Can you work these out from the model? Positions are in its coordinate system, mm. Face numbers are marked on the shaded views. Give positions to 0.01 mm unless a question says otherwise; leave off trailing zeros. Loops run counter-clockwise (first coordinate to the right, second up) from the corner with the lowest first, then second, coordinate; pieces in that order, holes last.
from build123d import *

# Parameters (mm, degrees)
BOSS_EXTRUDE1_DEPTH       = 2.54
F_3_0MM_DOWEL_HOLE1_D     = 3
F_3_0MM_DOWEL_HOLE1_DEPTH = 7.999984
F_3_0MM_DOWEL_HOLE1_TIP   = 0.901290929


with BuildPart() as part:
    # Sketch1 → Boss-Extrude1 (new body)
    with BuildSketch(Plane(origin=(0, 0, 0), x_dir=(1, 0, 0), z_dir=(0, 1, 0))):
        Polygon((59.944, 42.386808891), (42.386808891, 59.944), (17.557191109, 59.944), (0, 42.386808891), (0, 17.557191109), (17.557191109, 0), (42.386808891, 0), (59.944, 17.557191109), align=None)
        Polygon((4.468072616, 46.495671263), (6.26412384, 44.699620039), (15.244379961, 53.67987616), (13.448328737, 55.475927384), align=None, mode=Mode.SUBTRACT)
        Polygon((53.67987616, 44.699620039), (44.699620039, 53.67987616), (46.495671263, 55.475927384), (55.475927384, 46.495671263), align=None, mode=Mode.SUBTRACT)
    extrude(amount=BOSS_EXTRUDE1_DEPTH)

    # Ø3.0mm Dowel Hole1
    with Locations(Plane(origin=(0, 2.54, 0), x_dir=(1, 0, 0), z_dir=(0, 1, 0))):
        with Locations((2.9, 18.758410439), (57.044, 18.758410439), (2.9, 41.18558956), (57.044, 41.185589561), (18.758410439, 57.044), (41.185589561, 57.044)):
            Hole(F_3_0MM_DOWEL_HOLE1_D / 2, depth=F_3_0MM_DOWEL_HOLE1_DEPTH)
            with Locations((0, 0, -(F_3_0MM_DOWEL_HOLE1_DEPTH + F_3_0MM_DOWEL_HOLE1_TIP / 2))):  # 118° drill point
                Cone(0, F_3_0MM_DOWEL_HOLE1_D / 2, F_3_0MM_DOWEL_HOLE1_TIP, mode=Mode.SUBTRACT)


solid = part.part
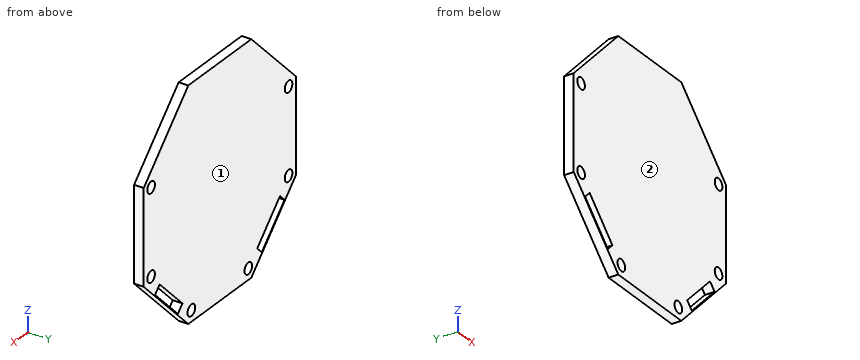
(1) Please list where these lines run through material, in increasing order: probe 1 along Z at (x, y) = (2.9, 1.4); probe 2 along X at (y, z) = (2.4, -46); probe 3 along X at (y, z) = (2.2, -52).
Returned:
probe 1: z = -45.29 to -42.69, -39.69 to -20.26, -17.26 to -14.66
probe 2: x = 3.61 to 4.96, 7.56 to 52.38, 54.98 to 56.33
probe 3: x = 9.61 to 9.97, 13.56 to 46.38, 49.97 to 50.33
(2) Suppose I cut it at C-C on x = 52. List the corners of the cut face in (y, z) for me, plus the area to 3 significant figures.
Returned:
outline: (0, -50.33) - (2.54, -50.33) - (2.54, -49.97) - (0, -49.97) - close; (0, -46.38) - (2.54, -46.38) - (2.54, -9.61) - (0, -9.61) - close
area: 94.3 mm2
(3) Thinking about a two-plate mould opening in Y: for the marked faces 1 and 2, which applies, pulls with the +Y half, pulls with the -Y half, needs draft (parallel to the pull), parting line crosses it, or undercut?
Returned:
face 1: pulls with the +Y half
face 2: pulls with the -Y half
(4) Suppose I cut it at B-B on z = -53. List the corners of the cut face in (x, y) for me, plus the area to 3 significant figures.
Returned:
outline: (10.61, 0) - (10.97, 0) - (10.97, 2.54) - (10.61, 2.54) - close; (14.56, 0) - (45.38, 0) - (45.38, 2.54) - (14.56, 2.54) - close; (48.97, 0) - (49.33, 0) - (49.33, 2.54) - (48.97, 2.54) - close
area: 80.1 mm2
(5) Suppose I cut it at D-D on y = 1.1. Give the number of separate pieces and of enclosed holes in the cut face, plus the area to 3 significant figures.
Returned:
separate pieces: 1
enclosed holes: 8
area: 2,870 mm2
(6) Suppose I cut it at A-A on x = 2.9. List the corners of the cut face in (y, z) for me.
Returned:
outline: (0, -45.29) - (2.54, -45.29) - (2.54, -42.69) - (0, -42.69) - close; (0, -39.69) - (2.54, -39.69) - (2.54, -20.26) - (0, -20.26) - close; (0, -17.26) - (2.54, -17.26) - (2.54, -14.66) - (0, -14.66) - close
(7) Will these pins go through, and if not, where does the flat tip stop? P1, Ø1, axis at y = 2, z = -10.5, coming from the +X side; P2, Ø1.5, axis at x = 16, y = 1, coming from the +Z side; P3, Ø1, axis at x = 47, y = 0.5, coming from the -Z side.
Returned:
P1: stops at x = 53.39
P2: stops at z = -0.81
P3: stops at z = -55.83
